Input: dimensioned drawing with shaded views. Units: mm. Origin: part minimum x, y, z. A direction names the side the tool comes from. Give positions to 0.01 mm unless a question says otherwise; leave off trailing zeros. Write each loop counter-clockwise with the first axis right and the second up, starting at its lowest first coordinate (ties: lowest second). Pieces come first, ordered by that corner, then holes. Notation, with made-up numbers: (-39, 14) -> (-28, 14) arc R20 ccw to (-28, 38) -> close; hole circle Ø10 at (69.5, 87.25). An arc over 180 degrees is marked (long way). Return JSON: item names as keys, results as strings. Group by question number.
Item 1: Section D-D, the plane x = 16.25. Return loops of the section in (y, z).
Item 2: Section C-C, the plane y = 7. Return loops of the section in (x, z).
Item 3: Section A-A, the plane y = 13.75. Return loops of the section in (x, z).
Item 4: Section B-B, the plane z = 57.5. Return loops of the section in (x, y).
Item 5: Line query: line 1 (Y direction, x = 1.45, z = 9.5); line 2 (X direction, y = 14.75, z = 59.5). Output: solid intervals per line, ascending. Write a range as [from, to].
Item 6: Pin query (flat end, axial travel): P1, Ø4, axis at y = 3.5, z = 59.5, coming from the -X side; P2, Ø4, axis at y = 15, z = 62, coming from the +X side; P3, Ø2, axis at x = 13, z = 17, coming from the +Y side. Return the tip coordinate at first contact, or that it passes through.
Item 7: Set-up query: the marked faces 1 and 2. Return all of +Z, -Z, +X, -X, +Y, -Y with unobstructed straight access to the full face (end or side cutting, diameter ignored); none if empty.
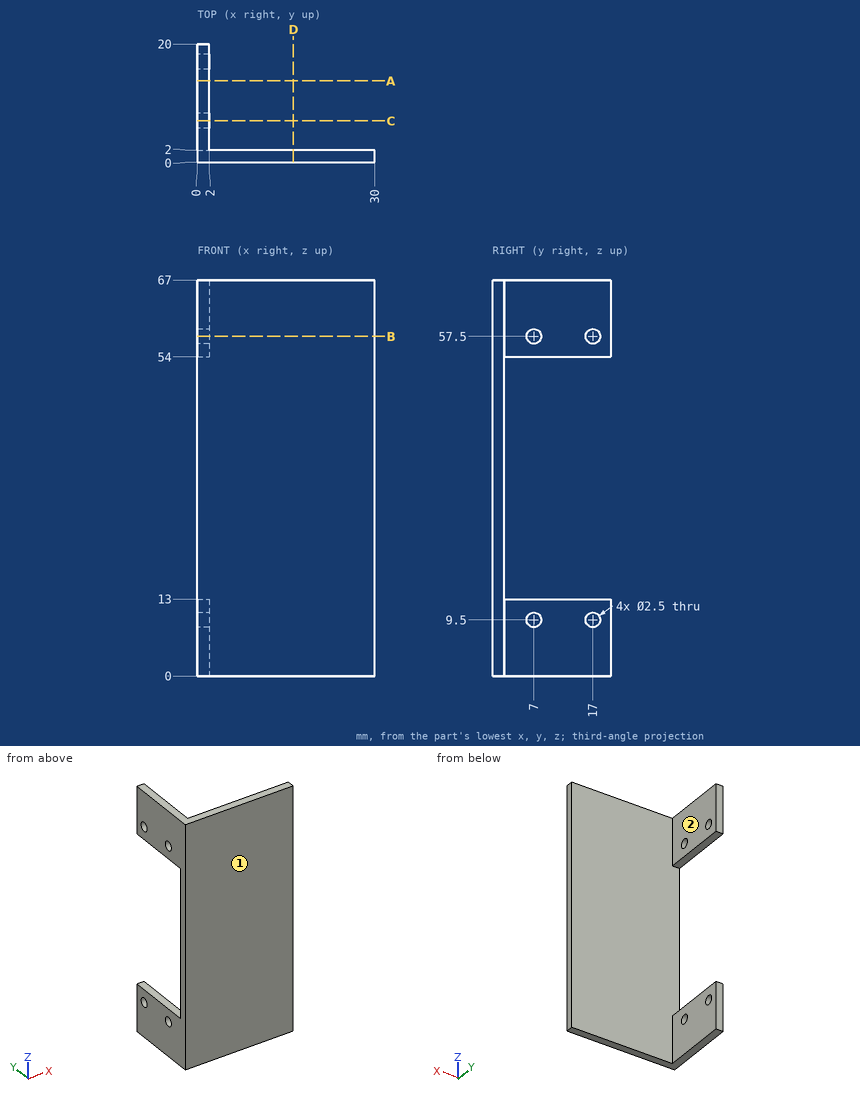
Answer below:
{
 "1": {"outline": "(0, 0) -> (2, 0) -> (2, 67) -> (0, 67) -> close"},
 "2": {"outline": "(0, 0) -> (2, 0) -> (2, 8.25) -> (0, 8.25) -> close; (0, 10.75) -> (2, 10.75) -> (2, 13) -> (0, 13) -> close; (0, 54) -> (2, 54) -> (2, 56.25) -> (0, 56.25) -> close; (0, 58.75) -> (2, 58.75) -> (2, 67) -> (0, 67) -> close"},
 "3": {"outline": "(0, 0) -> (2, 0) -> (2, 13) -> (0, 13) -> close; (0, 54) -> (2, 54) -> (2, 67) -> (0, 67) -> close"},
 "4": {"outline": "(0, 0) -> (30, 0) -> (30, 2) -> (2, 2) -> (2, 5.75) -> (0, 5.75) -> close; (0, 8.25) -> (2, 8.25) -> (2, 15.75) -> (0, 15.75) -> close; (0, 18.25) -> (2, 18.25) -> (2, 20) -> (0, 20) -> close"},
 "5": {"line 1": "y = [0, 5.75], [8.25, 15.75], [18.25, 20]", "line 2": "x = [0, 2]"},
 "6": {"P1": "stops at x = 0", "P2": "stops at x = 2", "P3": "stops at y = 2"},
 "7": {"face 1": "+Z, -Z, +X, -X, -Y", "face 2": "+Z, -Z, +X, +Y"}
}
